Geometry check sheet. Reference: the model listing, model coordinates, mm. Give positions to 0.01 mm unless a question says otherwise; leave off trailing zeros. Write each loop counter-clockwise with the first axis right and the second up, starting at its lowest first coordinate (ties: lowest second). Pieces come first, ordered by that corner, then holes. Notation, with made-up numbers: (-3.5, 10.25) -> (25.5, 10.25) arc R22 cw to (25.5, 33.25) -> close; hole circle Ø2 at (8, -33). An arc over 180 degrees is marked (long way). Use a Markdown table: item, result. Add a question column.
from build123d import *

# Parameters (mm, degrees)
ESQUISSE2_R        = 1.5
BOSS_EXTRU_1_DEPTH = 4


with BuildPart() as part:
    # Esquisse2 → Boss.-Extru.1 (new body)
    with BuildSketch(Plane(origin=(0, 0, 0), x_dir=(1, 0, 0), z_dir=(0, 1, 0))):
        with BuildLine():
            Line((0, 0), (28, 0))
            Line((28, 0), (28, -160))
            Line((28, -160), (172, -160))
            Line((172, -160), (172, 0))
            Line((172, 0), (200, 0))
            ThreePointArc((200, 0), (100, 40), (0, 0))
        make_face()
        with Locations(Location((44.519959109, -134.645808038, 0), (0, 0, 270))):
            Circle(ESQUISSE2_R, mode=Mode.SUBTRACT)
        with Locations(Location((44.519959109, -150.668405535, 0), (0, 0, 270))):
            Circle(ESQUISSE2_R, mode=Mode.SUBTRACT)
        with Locations(Location((155.480040891, -150.668405535, 0), (0, 0, 90))):
            Circle(ESQUISSE2_R, mode=Mode.SUBTRACT)
        with Locations(Location((155.480040891, -134.645808038, 0), (0, 0, 90))):
            Circle(ESQUISSE2_R, mode=Mode.SUBTRACT)
        with Locations(Location((75.412395646, 0, 0), (0, 0, 270))):
            Circle(ESQUISSE2_R, mode=Mode.SUBTRACT)
        with Locations(Location((124.587604354, 0, 0), (0, 0, 90))):
            Circle(ESQUISSE2_R, mode=Mode.SUBTRACT)
        with BuildLine():
            ThreePointArc((185.657545612, 9.025506382), (100.445588201, 35.657742009), (15.23363079, 9.025506382))
            ThreePointArc((15.23363079, 9.025506382), (14.672053701, 5.931560858), (17.765999225, 5.369983769))
            ThreePointArc((17.765999225, 5.369983769), (100.445588201, 31.210750277), (183.125177177, 5.369983769))
            ThreePointArc((183.125177177, 5.369983769), (186.219122701, 5.931560858), (185.657545612, 9.025506382))
        make_face(mode=Mode.SUBTRACT)
    extrude(amount=BOSS_EXTRU_1_DEPTH)


solid = part.part
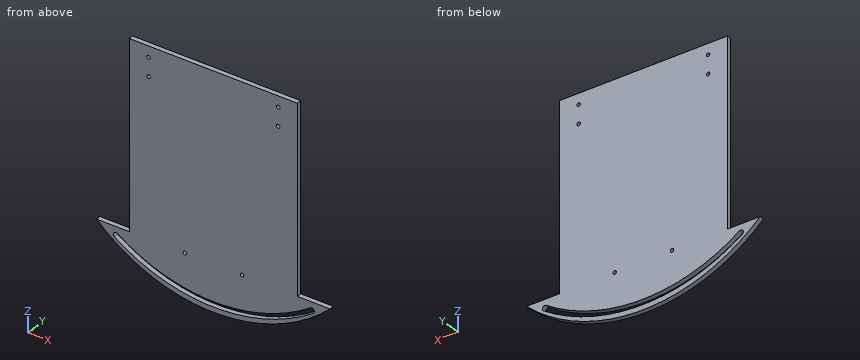
1) Material ranges on probe 1 along X at (y, z) = (2.45, -8); probe 2 along X at (y, z) = (3.8, 136); probe 3 along X at (y, z) = (3.8, 78.5), recorded low to high. Write a range as [from, to].
2) Sectioned sample at C-C, the plane z = 95.5. Enter the section's corners in (x, y), and give its area (3 significant figures).
3) Sectioned sample at D-D, the plane x = 150. Enter the section's corners in (y, z), and give its area (3 significant figures).
4) Sectioned sample at B-B, the plane y = 1.75. Enter the section's corners in (x, z).
5) Gauge pin test, flat ends, axial feed: P1, Ø2, axis at y = 2.5, z = 106, coming from the +X side; P2, Ø1.5, axis at y = 2, z = 22, coming from the -X side; P3, Ø1.2, axis at x = 183, y = 1.5, coming from the +Z side. Record the tip position at first contact, or that the pin passes through.
6) Sectioned sample at A-A, the plane x = 90. Enter the section's corners in (y, z).
Check values:
| question | item | result |
|---|---|---|
| 1 | probe 1 | [9.14, 14.43], [21.7, 179.19], [186.47, 190.86] |
| 1 | probe 2 | [28, 43.87], [45.17, 154.83], [156.13, 172] |
| 1 | probe 3 | [28, 172] |
| 2 | outline | (28, 0) -> (172, 0) -> (172, 4) -> (28, 4) -> close |
| 2 | area | 576 mm² |
| 3 | outline | (0, -31.11) -> (4, -31.11) -> (4, -27.21) -> (0, -27.21) -> close; (0, -22.49) -> (4, -22.49) -> (4, 160) -> (0, 160) -> close |
| 3 | area | 746 mm² |
| 4 | outline | (0, 0) arc R145 ccw to (200, 0) -> (172, 0) -> (172, 160) -> (28, 160) -> (28, 0) -> close; hole (15.23, -9.03) arc R149.64 ccw to (185.66, -9.03) arc R2.22 ccw to (183.13, -5.37) arc R145.19 cw to (17.77, -5.37) arc R2.22 ccw to start; hole circle Ø3 at (44.52, 134.65); hole circle Ø3 at (44.52, 150.67); hole circle Ø3 at (75.41, 0); hole circle Ø3 at (124.59, 0); hole circle Ø3 at (155.48, 134.65); hole circle Ø3 at (155.48, 150.67) |
| 5 | P1 | x = 172 |
| 5 | P2 | x = 28 |
| 5 | P3 | z = 0 |
| 6 | outline | (0, -39.65) -> (4, -39.65) -> (4, -35.29) -> (0, -35.29) -> close; (0, -30.83) -> (4, -30.83) -> (4, 160) -> (0, 160) -> close |
